Could you check a few things on this model? Use its own coordinates, in mm. A direction names the side the tool comes from. Round coordinates to 2 decimals unless told otherwise and drop trailing zeros. Order: outer loops, then holes, each group sorted by start corner. A loop starts at its lowest first (then second) coordinate and runs counter-clockwise, first axis right, second up. Notation, with made-up numbers: (69, -34.75) - (104, -34.75) arc R20 cw to (104, -18.75) - close; hole circle Ø8 at (-11, 30). An arc over 180 degrees is marked (long way). Return JSON: item names as keys, results as strings. Group by question number.
from build123d import *

# Parameters (mm, degrees)
BOSS_EXTRUDE1_DEPTH = 1
SKETCH2_W           = 1
SKETCH2_H           = 26
BOSS_EXTRUDE2_DEPTH = 43
CUT_EXTRUDE1_DEPTH  = 1
FILLET1_R           = 1


with BuildPart() as part:
    # Sketch1 → Boss-Extrude1 (new body)
    with BuildSketch(Plane(origin=(0, 0, 0), x_dir=(1, 0, 0), z_dir=(0, 1, 0))):
        with BuildLine():
            Line((-23, 13), (21, 13))
            ThreePointArc((21, 13), (22.414213562, 12.414213562), (23, 11))
            Line((23, 11), (23, -11))
            ThreePointArc((23, -11), (22.414213562, -12.414213562), (21, -13))
            Line((21, -13), (-23, -13))
            Line((-23, -13), (-23, 13))
        make_face()
        with BuildLine():
            Line((-4.5, 9), (4.5, 9))
            ThreePointArc((4.5, 9), (13.5, 0), (4.5, -9))
            Line((4.5, -9), (-4.5, -9))
            ThreePointArc((-4.5, -9), (-13.5, 0), (-4.5, 9))
        make_face(mode=Mode.SUBTRACT)
    extrude(amount=BOSS_EXTRUDE1_DEPTH)

    # Sketch2 → Boss-Extrude2 (add)
    with BuildSketch(Plane(origin=(0, 1, 0), x_dir=(1, 0, 0), z_dir=(0, 1, 0))):
        with Locations((-22.5, 0)):
            Rectangle(SKETCH2_W, SKETCH2_H)
    extrude(amount=BOSS_EXTRUDE2_DEPTH)

    # Sketch3 → Cut-Extrude1 (cut)
    with BuildSketch(Plane(origin=(-22, 0, 0), x_dir=(0, 0, -1), z_dir=(1, 0, 0))):
        with BuildLine():
            Line((-3.75, 22.5), (3.75, 22.5))
            ThreePointArc((3.75, 22.5), (5.75, 20.5), (3.75, 18.5))
            Line((3.75, 18.5), (-3.75, 18.5))
            ThreePointArc((-3.75, 18.5), (-5.75, 20.5), (-3.75, 22.5))
        make_face()
    extrude(amount=-CUT_EXTRUDE1_DEPTH, mode=Mode.SUBTRACT)

    # Fillet1
    fillet1_edges = [part.edges().sort_by_distance(p)[0] for p in [
        (-22.5, 44, -13),
        (-22.5, 44, 13),
    ]]
    fillet(fillet1_edges, radius=FILLET1_R)


solid = part.part
1) Will these pins go through, and if not, where does the flat tip stop? pin 1 (1 mm diameter, centred on y = 6, z = 0.5, fed in from +X); pin 2 (6 mm diameter, centred on x = -4, z = -7.5, fed in from +Y).
2) I want a section at B-B, the plane x = 2. List the corners of the cut face in (y, z) for me.
3) For faces 1 (the cylindrical face through (13.498, 0.493, -0.198)), 2 (the cylindrical face through (-22.49, 20.54, -5.75)), 3 (the flat face through (1, 1, 11)), which set-ups out of +Z, -Z, +X, -X, +Y, -Y let a thin tool reach every point of the face, with its end or its side?
4) I want a section at C-C, the plane z = 0. List the corners of the cut face in (x, y) for me.
5) I want a section at D-D, the plane z = -9.75. List the corners of the cut face in (x, y) for me, plus the area to 3 significant figures.
6) We'd pull the mould along X, two halves only. Please class faces 4 (the flat face through (-10.9, 0.7, -13)), 5 (the cylindrical face through (22.43, 0.49, 12.4)), 6 (the cylindrical face through (-13.498, 0.493, 0.198)): +X half, -X half, draft (parallel to the pull), parting line (faces both ways), or undercut.
7) I want a section at A-A, the plane y = 20.5. List the corners of the cut face in (x, z) for me, plus the area to 3 significant figures.
8) If I drill on line 1 along Y through (x, z) = (-8, -11.5); line 2 along X through (y, z) = (34.5, 8.5), over which ranges is the centre line in solid material (lowest first)? Write a range as from..to.
Outcome:
{
 "1": {"pin 1": "x = -22", "pin 2": "y = 1"},
 "2": {"outline": "(0, -13) - (1, -13) - (1, -9) - (0, -9) - close; (0, 9) - (1, 9) - (1, 13) - (0, 13) - close"},
 "3": {"face 1": "+Y, -Y", "face 2": "+X, -X", "face 3": "+Z, -Z, +X, +Y"},
 "4": {"outline": "(-23, 0) - (-13.5, 0) - (-13.5, 1) - (-22, 1) - (-22, 18.5) - (-23, 18.5) - close; (-23, 22.5) - (-22, 22.5) - (-22, 44) - (-23, 44) - close; (13.5, 0) - (23, 0) - (23, 1) - (13.5, 1) - close"},
 "5": {"outline": "(-23, 0) - (23, 0) - (23, 1) - (-22, 1) - (-22, 44) - (-23, 44) - close", "area": "89.0 mm^2"},
 "6": {"face 4": "draft", "face 5": "+X half", "face 6": "undercut"},
 "7": {"outline": "(-23, -13) - (-22, -13) - (-22, -5.75) - (-23, -5.75) - close; (-23, 5.75) - (-22, 5.75) - (-22, 13) - (-23, 13) - close", "area": "14.5 mm^2"},
 "8": {"line 1": "0..1", "line 2": "-23..-22"}
}
